Source: three-view drawing plus pictorial views. Frame: mm from the lowest corner of the part. Round coordinates to 2 decimals unless told otherwise and drop trailing zeros. Order: outer loops, then holes, each group sorted by start corner. A loop starts at its lowest first (then second) coordinate and runs counter-clockwise, first axis right, second up. Notation, with made-up numbers: (29, 43.25) - (68, 43.25) arc R13 cw to (68, 51.25) - close; hole circle Ø5 at (-5.5, 76). An arc over 180 degrees is marked (long way). Use one line per item in the form item = value. Start each with the question number.
Q1. Cut plane C-C, the plane y = 7.5. Return the cut outline in (x, z), and give its area (3 significant figures).
Q2. Ray query, line 1 (Y direction, x = 42.5, z = 25); line 2 (X direction, y = 3.5, z = 33.5) (1 decimal); line 3 (Z direction, x = 39.5, y = 5) (1 decimal). Return the intervals inside material, ascending. Write a range as [from, to].
Q3. Pin query (flat end, axial travel): pin 1 Ø1 at (y, z) = (6.5, 36) entering from -X; pin 2 Ø3 at (x, y) = (32, 3.5) entering from +Z; pin 3 Ø2 at (x, y) = (27, 8) entering from -Z. Return the tip coordinate at first contact, or that it passes through.
Q4. Cut plane B-B, the plane z = 25. Return the cut outline in (x, y).
Q5. Cut plane D-D, the plane y = 2.25. Return the cut outline in (x, z).
Q6. Cut plane A-A, the plane x = 25. Return the cut outline in (y, z), and give its area (3 significant figures).
Q7. Draft query along Z for the marked faces 1, 2 and 3. Return one class per face: released by +Z, released by -Z, zero draft, split by the parting line, or undercut.
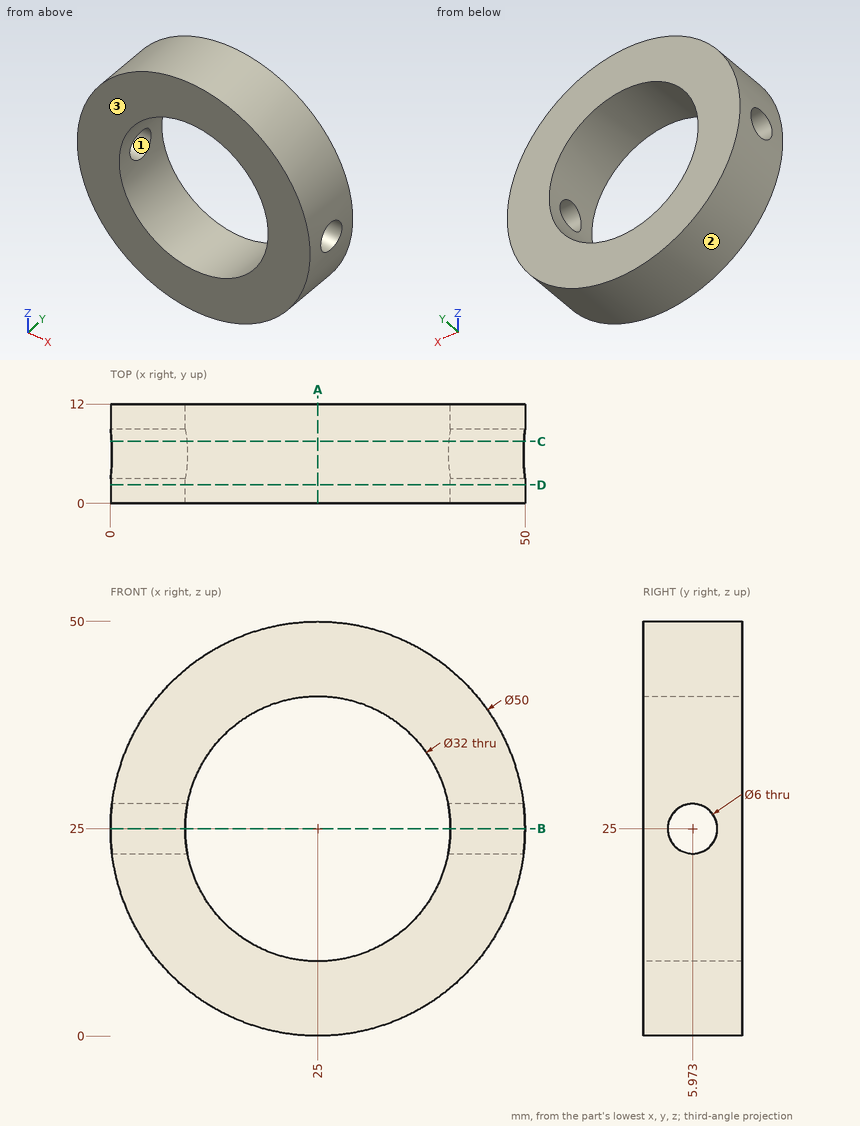
Completed:
q1.outline = (0.13, 22.42) arc R25 ccw to (49.87, 22.42) - (40.79, 22.42) arc R16 cw to (9.21, 22.42) - close; (0.13, 27.58) - (9.21, 27.58) arc R16 cw to (40.79, 27.58) - (49.87, 27.58) arc R25 ccw to start
q1.area = 1,070 mm2
q2.line_1 = [0, 2.97], [8.97, 12]
q2.line_2 = [1.5, 11.4], [38.6, 48.5]
q2.line_3 = [4.6, 18.2], [31.8, 45.4]
q3.pin_1 = 2.31
q3.pin_2 = 49.39
q3.pin_3 = 0.02
q4.outline = (0, 0) - (9, 0) - (9, 2.97) - (0, 2.97) - close; (0, 8.97) - (9, 8.97) - (9, 12) - (0, 12) - close; (41, 0) - (50, 0) - (50, 2.97) - (41, 2.97) - close; (41, 8.97) - (50, 8.97) - (50, 12) - (41, 12) - close
q5.outline = circle Ø50 at (25, 25); hole circle Ø32 at (25, 25)
q6.outline = (0, 0) - (12, 0) - (12, 9) - (0, 9) - close; (0, 41) - (12, 41) - (12, 50) - (0, 50) - close
q6.area = 216 mm2
q7.face_1 = undercut
q7.face_2 = split by the parting line
q7.face_3 = zero draft
